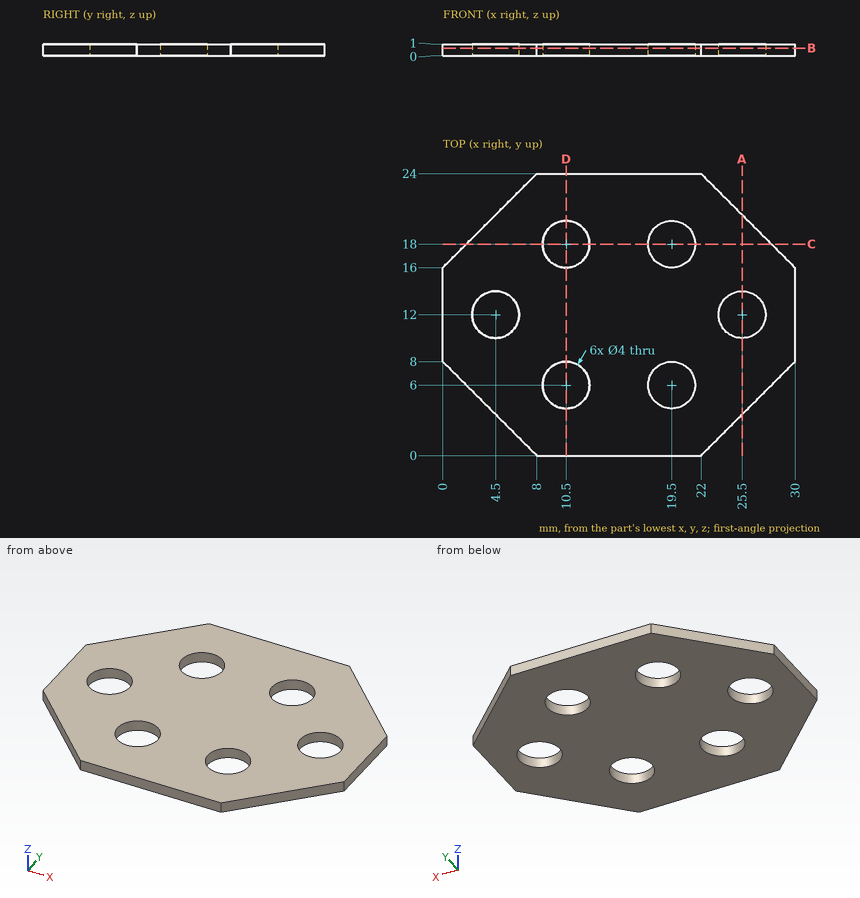
The drawing under review shows one solid part. Ordinate dimensions are in mm from its lowest x, y, z. Round coordinates to 2 decimals unless told otherwise and drop trailing zeros. Write each loop counter-clockwise with the first axis right and the second up, starting at its lowest first coordinate (ties: lowest second). Pieces come first, ordered by that corner, then holes.
(1) Wall thickness on L1, parallel to Y at x = 19.5, z = 0.6; L2, parallel to Y at x = 12, z = 0.1; L3, parallel to X at y = 12.5, z = 0.2: over which ranges is each line inside the solid? List them lowest first.
(2) We need section C-C on y = 18. Give the boundary of the cut face in (x, z).
(3) We need section B-B on z = 0.65. Give the boundary of the cut face in (x, y).
(4) We need section D-D on x = 10.5. Give the boundary of the cut face in (y, z).
(5) Insertion check: pin 1 (3 mm diameter, centred on x = 4.5, y = 12, fed in from -Z) (1 decimal). The pin has a flat end and moves straight along its axis. Give the tip position at first contact, or say it passes through.
(6) We need section A-A on x = 25.5. Give the boundary of the cut face in (y, z).
Findings below:
1. L1: y = 0 to 4, 8 to 16, 20 to 24
1. L2: y = 0 to 4.68, 7.32 to 16.68, 19.32 to 24
1. L3: x = 0 to 2.56, 6.44 to 23.56, 27.44 to 30
2. outline: (2, 0) - (8.5, 0) - (8.5, 1) - (2, 1) - close; (12.5, 0) - (17.5, 0) - (17.5, 1) - (12.5, 1) - close; (21.5, 0) - (28, 0) - (28, 1) - (21.5, 1) - close
3. outline: (0, 8) - (8, 0) - (22, 0) - (30, 8) - (30, 16) - (22, 24) - (8, 24) - (0, 16) - close; hole circle Ø4 at (4.5, 12); hole circle Ø4 at (10.5, 6); hole circle Ø4 at (10.5, 18); hole circle Ø4 at (19.5, 6); hole circle Ø4 at (19.5, 18); hole circle Ø4 at (25.5, 12)
4. outline: (0, 0) - (4, 0) - (4, 1) - (0, 1) - close; (8, 0) - (16, 0) - (16, 1) - (8, 1) - close; (20, 0) - (24, 0) - (24, 1) - (20, 1) - close
5. pin 1: passes through
6. outline: (3.5, 0) - (10, 0) - (10, 1) - (3.5, 1) - close; (14, 0) - (20.5, 0) - (20.5, 1) - (14, 1) - close
